Could you check a few things on this drawing? It's one solid part, dimensions in mm from its lowest x, y, z. Give positions to 0.01 mm unless a question says otherwise; leave off trailing zeros. Loops run counter-clockwise (first coordinate to the right, second up) from the corner with the lowest first, then second, coordinate; pieces in that order, holes last. Notation, with made-up numbers: M 47,74 L 103,74 A12 cw 103,94 Z; hole C -23.5,6 d4. An arc over 180 degrees is marked long. One line per item, written item: value. Start each with the question number.
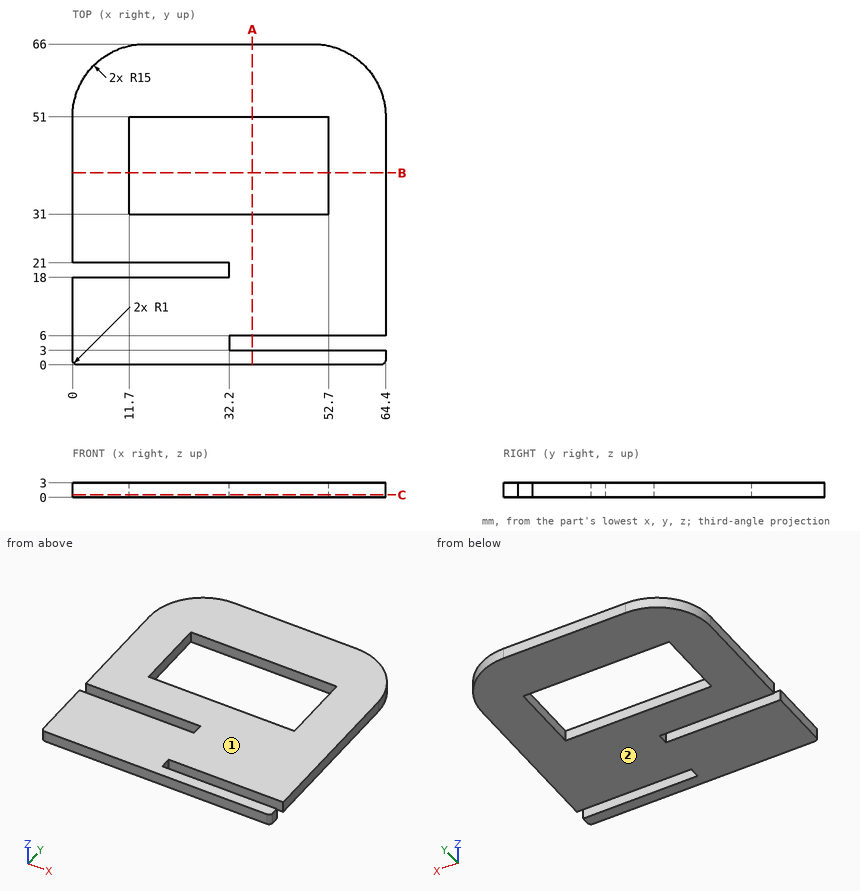
Q1. I need wall thicknesses on line 1 along Y through (x, z) = (16.5, 0.8); line 2 along Y through (x, z) = (40.5, 2.05); line 3 along X through (y, z) = (34.5, 1.2). Which ranges of each line are inside material? Lowest first, please.
Q2. If we section it at B-B, the plane y = 39.5: Write out the boundary of the cut face in (x, z), plus the area to 3 significant figures.
Q3. For P1, Ø1.5, axis at x = 52, z = 1, coming from the +Y side; P2, Ø0.9, axis at y = 39, z = 1, coming from the -X side; P3, Ø1.5, axis at y = 4.5, z = 1.5, coming from the +X side, each with a flat end and sliding along its axis, tell me the tip position at first contact or that it passes through.
Q4. If we section it at A-A, the plane x = 37: Write out the boundary of the cut face in (y, z), plus the area to 3 significant figures.
Q5. If we section it at C-C, the plane z = 0.55: Write out the boundary of the cut face in (x, y), plus the area to 3 significant figures.
Q6. If we mould it in two halves opening along Z, with no side actions, what happens to the marked faces 1 and 2? For each: released by +Z, released by -Z, zero draft, split by the parting line, or undercut.
Response:
1. line 1: 0 to 18, 21 to 31, 51 to 66
1. line 2: 0 to 3, 6 to 31, 51 to 66
1. line 3: 0 to 11.7, 52.7 to 64.4
2. outline: M 0,0 L 11.7,0 L 11.7,3 L 0,3 Z; M 52.7,0 L 64.4,0 L 64.4,3 L 52.7,3 Z
2. area: 70.2 mm^2
3. P1: y = 65.89
3. P2: x = 0
3. P3: x = 32.2
4. outline: M 0,0 L 3,0 L 3,3 L 0,3 Z; M 6,0 L 31,0 L 31,3 L 6,3 Z; M 51,0 L 66,0 L 66,3 L 51,3 Z
4. area: 129 mm^2
5. outline: M 0,1 A1 ccw 1,0 L 63.4,0 A1 ccw 64.4,1 L 64.4,3 L 32.2,3 L 32.2,6 L 64.4,6 L 64.4,51 A15 ccw 49.4,66 L 15,66 A15 ccw 0,51 L 0,21 L 32.2,21 L 32.2,18 L 0,18 Z; hole M 11.7,31 L 52.7,31 L 52.7,51 L 11.7,51 Z
5. area: 3,140 mm^2
6. face 1: released by +Z
6. face 2: released by -Z
